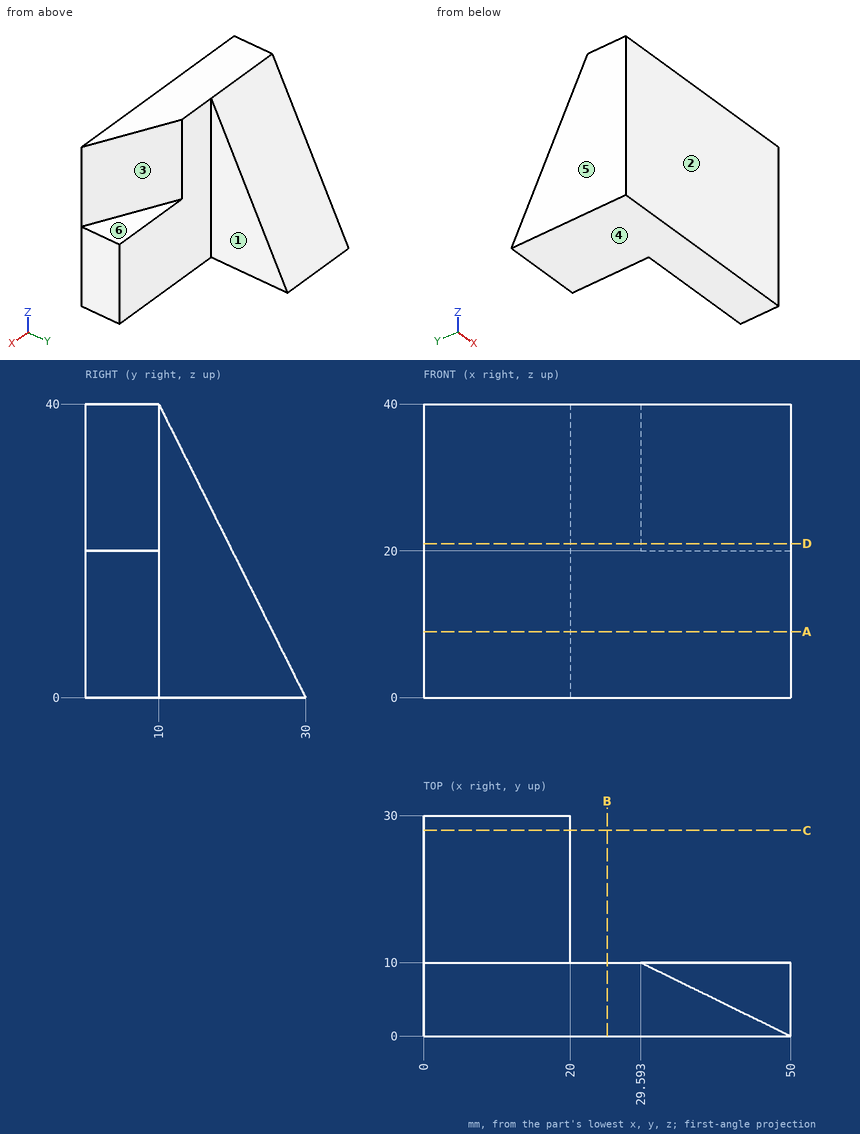
Job drawing, mm, ordinate dimensions from the low corner. One solid piece. A direction names the side the tool comes from. Round coordinates to 2 decimals unless told otherwise and drop trailing zeros. Write each loop counter-clockwise with the first axis right and the second up, starting at its lowest first coordinate (ties: lowest second). Pieces come first, ordered by that corner, then holes. Notation, with made-up numbers: (-23, 7) -> (-18, 7) arc R8 cw to (-18, 15) -> close; hole circle Ø2 at (-38, 78). An arc over 180 degrees is marked (long way). Answer as CSV lines item,"result".
1. Pin check, flat tips, straight feed: pin 1 Ø10 at (x, z) = (25, 7.5) entering from -Y; pin 2 Ø1 at (x, z) = (27, 19.5) entering from +Y; pin 3 Ø10 at (y, z) = (6.5, 34.5) entering from +X; pin 4 Ø6 at (y, z) = (15.5, 20.5) entering from +X. Stop position of each tip, or through.
Resolved:
pin 1,"y = 0"
pin 2,"y = 10"
pin 3,"x = 46.94"
pin 4,"x = 20"
2. Slice it at D-D, the plane z = 21. List the corners of the cut face in (x, y), plus the area to 3 significant figures.
Resolved:
outline,"(0, 0) -> (50, 0) -> (29.59, 10) -> (20, 10) -> (20, 19.5) -> (0, 19.5) -> close"
area,"588 mm²"
3. Tool access for the marked faces 1, 2 and 3: list every direction of +Z, -Z, +X, -X, +Y, -Y with a clear straight run to the whole face (end or side of a thin tool).
Resolved:
face 1,"+Z, -Z, +X, +Y"
face 2,"+Z, -Z, +X, -X, -Y"
face 3,"+Z, +X, +Y"
4. Mould opens along Z. For the marked faces 4, 5 and 6 say: +Z half, -Z half, draft (parallel to the pull), parting line (faces both ways), or undercut.
Resolved:
face 4,"-Z half"
face 5,"draft"
face 6,"+Z half"
5. Slice it at B-B, the plane x = 25. List the corners of the cut face in (y, z).
Resolved:
outline,"(0, 0) -> (10, 0) -> (10, 40) -> (0, 40) -> close"
6. Slice it at A-A, the plane z = 9. List the corners of the cut face in (x, y), plus the area to 3 significant figures.
Resolved:
outline,"(0, 0) -> (50, 0) -> (50, 10) -> (20, 10) -> (20, 25.5) -> (0, 25.5) -> close"
area,"810 mm²"
7. Slice it at C-C, the plane y = 28. List the corners of the cut face in (x, z), plus the area to 3 significant figures.
Resolved:
outline,"(0, 0) -> (20, 0) -> (20, 4) -> (0, 4) -> close"
area,"80.0 mm²"
8. Drill centre lines: line 1 (X direction, y = 18.5, z = 5.5); line 2 (Y direction, x = 40, z = 8). Where is each one in solid material? Low to high.
Resolved:
line 1,"0 to 20"
line 2,"0 to 10"
